from build123d import *

# Parameters (mm, degrees)
REVOLVE2_ANGLE           = 7.5
REVOLVE2_OTHER_WAY_ANGLE = 7.5
CUT_EXTRUDE1_DEPTH       = 16.24
CUT_EXTRUDE1_DEPTH_BACK  = 16.24


with BuildPart() as part:
    # Sketch1 → Revolve1 (revolve)
    with BuildSketch(Plane.XY):
        with BuildLine():
            Line((0, 12.7), (-1.27, 12.7))
            Line((-1.27, 12.7), (-1.27, 13.97))
            Line((-1.27, 13.97), (0, 13.97))
            ThreePointArc((0, 13.97), (9.878281733, 9.878281733), (13.97, 0))
            Line((13.97, 0), (12.7, 0))
            ThreePointArc((12.7, 0), (8.980256121, 8.980256121), (0, 12.7))
        make_face()
    revolve(axis=Axis((-1.27, 13.97, 0), (0, -1, 0)))

    # Sketch3 → Revolve2 (revolve)
    with BuildSketch(Plane.XY):
        with BuildLine():
            Line((0, 13.97), (50.8, 13.97))
            Line((50.8, 13.97), (50.8, 0))
            Line((50.8, 0), (13.97, 0))
            ThreePointArc((13.97, 0), (9.878281733, 9.878281733), (0, 13.97))
        make_face()
    revolve(axis=Axis((-1.27, 13.97, 0), (0, -1, 0)), revolution_arc=REVOLVE2_ANGLE)

    # Sketch3 → Revolve2 other way (revolve)
    with BuildSketch(Plane.XY):
        with BuildLine():
            Line((0, 13.97), (50.8, 13.97))
            Line((50.8, 13.97), (50.8, 0))
            Line((50.8, 0), (13.97, 0))
            ThreePointArc((13.97, 0), (9.878281733, 9.878281733), (0, 13.97))
        make_face()
    revolve(axis=Axis((-1.27, 13.97, 0), (0, 1, 0)), revolution_arc=REVOLVE2_OTHER_WAY_ANGLE)

    # Sketch4 → Cut-Extrude1 (cut, two sides)
    with BuildSketch(Plane.XY) as cut_extrude1_sk:
        with BuildLine():
            Line((50.354533932, 13.97), (57.446880617, 13.97))
            Line((57.446880617, 13.97), (57.446880617, -0.511564319))
            Line((57.446880617, -0.511564319), (50.354533932, 0))
            Line((50.354533932, 0), (46.321742301, 0))
            Line((46.321742301, 0), (48.767033932, 4.235369343))
            ThreePointArc((48.767033932, 4.235369343), (47.179533932, 6.985), (48.767033932, 9.734630657))
            Line((48.767033932, 9.734630657), (46.321742301, 13.97))
            Line((46.321742301, 13.97), (50.354533932, 13.97))
        make_face()
    extrude(amount=CUT_EXTRUDE1_DEPTH, mode=Mode.SUBTRACT)
    extrude(cut_extrude1_sk.sketch, amount=-CUT_EXTRUDE1_DEPTH_BACK, mode=Mode.SUBTRACT)


solid = part.part
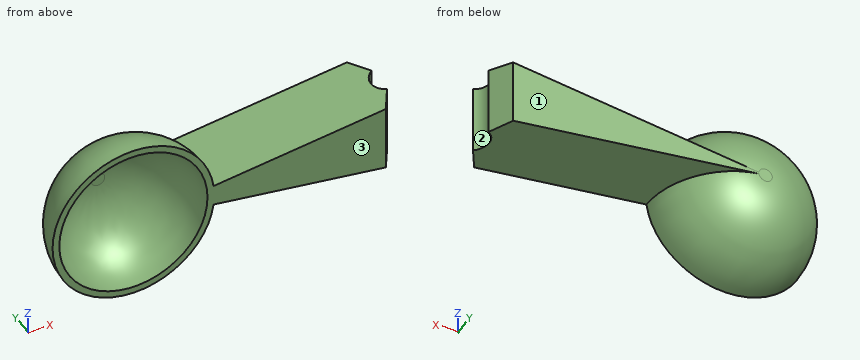
Read the model definition and answer for the solid it produces. Units are mm, in the model's axes. Face numbers are marked on the shaded views. Coordinates: 2 decimals unless noted, no trailing zeros. Write each loop counter-clockwise with the first axis right and the second up, starting at its lowest first coordinate (ties: lowest second). Pieces come first, ordered by that corner, then holes. Notation, with made-up numbers: M 29.5,17.25 L 43.5,17.25 A11 ccw 43.5,21.25 Z; hole C 13,-28.5 d4. An arc over 180 degrees is marked long. Use a Markdown table: item, result.
Q1. Each of these flat-tipped pins is pushed along its axis until it touches: pin 1 Ø8 at (x, z) = (0, -1.5) entering from -Y; pin 2 Ø6 at (y, z) = (2.5, 9.5) entering from -X; pin 3 Ø4 at (x, y) = (12, 3.5) entering from +Z. Where does it stop, or does it pass through?
Answer block:
| item | result |
|---|---|
| pin 1 | stops at y = 11.8 |
| pin 2 | stops at x = -14.89 |
| pin 3 | stops at z = 9.7 |
Q2. Straight lines are drawn through the part: L1, parallel to X at y = 5, z = -11.5; L2, parallel to Z at x = -12.5, y = 6.5; L3, parallel to Z at x = 3, y = 8.5. For each, find the intervals that lie inside material, in ascending order. Write a range as [from, to].
Answer block:
| item | result |
|---|---|
| L1 | x = [-9.79, -7.21], [4.67, 7.25] |
| L2 | z = [-7.73, -4.72], [4.72, 7.73] |
| L3 | z = [-11.6, -9.82], [9.82, 11.6] |
Q3. Determine the mould class of the marked faces 1, 2 and 3 for opening direction Y: released by +Y, released by -Y, zero draft, split by the parting line, or undercut.
Answer block:
| item | result |
|---|---|
| face 1 | released by +Y |
| face 2 | undercut |
| face 3 | released by -Y |
Q4. The part is cut by section A-A, the plane x = 33. Write down the section's boundary in (y, z).
Answer block:
| item | result |
|---|---|
| outline | M 0,-4.51 L 13.97,-4.51 L 13.97,4.51 L 0,4.51 Z |
